```python
from build123d import *

# Parameters (mm, degrees)
SKETCH_1_W          = 82
SKETCH_1_H          = 40
EXTRUDE_1_DEPTH     = 8
SKETCH_3_W          = 10
SKETCH_3_H          = 5
EXTRUDE_3_DEPTH     = 20
SKETCH_4_R          = 1.5
CUT_EXTRUDE_1_DEPTH = 47


with BuildPart() as part:
    # 草图1 → 凸台-拉伸1 (new body)
    with BuildSketch(Plane.XY):
        with Locations((15.184210526, 10.907894737)):
            Rectangle(SKETCH_1_W, SKETCH_1_H)
        with BuildLine():
            Line((46.184210526, -1.592105263), (36.184210526, -1.592105263))
            ThreePointArc((36.184210526, -1.592105263), (33.684210526, 0.907894737), (36.184210526, 3.407894737))
            Line((36.184210526, 3.407894737), (46.184210526, 3.407894737))
            ThreePointArc((46.184210526, 3.407894737), (48.684210526, 0.907894737), (46.184210526, -1.592105263))
        make_face(mode=Mode.SUBTRACT)
        with BuildLine():
            Line((46.184210526, 18.407894737), (36.184210526, 18.407894737))
            ThreePointArc((36.184210526, 18.407894737), (33.684210526, 20.907894737), (36.184210526, 23.407894737))
            Line((36.184210526, 23.407894737), (46.184210526, 23.407894737))
            ThreePointArc((46.184210526, 23.407894737), (48.684210526, 20.907894737), (46.184210526, 18.407894737))
        make_face(mode=Mode.SUBTRACT)
    extrude(amount=EXTRUDE_1_DEPTH)

    # 草图3 → 凸台-拉伸3 (add)
    with BuildSketch(Plane.XY.offset(8)):
        with Locations((-20.815789474, 28.407894737)):
            Rectangle(SKETCH_3_W, SKETCH_3_H)
        with Locations((-20.815789474, -6.592105263)):
            Rectangle(SKETCH_3_W, SKETCH_3_H)
        with Locations((-20.815789474, 10.907894737)):
            Rectangle(SKETCH_3_W, SKETCH_3_H)
    extrude(amount=EXTRUDE_3_DEPTH)

    # 草图4 → 切除-拉伸1 (cut)
    with BuildSketch(Plane(origin=(0, 30.907894737, 0), x_dir=(1, 0, 0), z_dir=(0, 1, 0))):
        with Locations(Location((-20.815789474, -18, 0), (0, 0, 270))):
            Circle(SKETCH_4_R)
    extrude(amount=-CUT_EXTRUDE_1_DEPTH, mode=Mode.SUBTRACT)


solid = part.part
```
Geometry check sheet. Reference: the model listing, model coordinates, mm. A direction names the side the tool comes from. Give positions to 0.01 mm unless a question says otherwise; leave off trailing zeros. Write each loop counter-clockwise with the first axis right and the second up, starting at its lowest first coordinate (ties: lowest second). Pieces come first, ordered by that corner, then holes.
1) Section check C-C, the plane z = 18. Record the boundary of the cut face in (x, y), and give its area (3 significant figures).
2) Section check A-A, the plane z = 24.25. Record the boundary of the cut face in (x, y), and give its area (3 significant figures).
3) Gauge pin test, flat ends, axial feed: pin 1 (3 mm diameter, centred on x = 25, y = 10, fed in from -Z); pin 2 (4 mm diameter, centred on y = -6, z = 17, fed in from +X); pin 3 (5 mm diameter, centred on x = 41, y = 5.5, fed in from +Z). Record the tip position at first contact, or that the pin passes through.
4) Section check D-D, the plane y = 21.5. Record the boundary of the cut face in (x, z).
5) Material ranges on L1, parallel to Y at x = 46, z = 1.75; L2, parallel to X at y = 11.15, z = 18; L3, parallel to Z at x = -17, y = 6, recorded low to high.
6) Section check B-B, the plane x = 41. Record the boundary of the cut face in (y, z), and give its area (3 significant figures).
7) Access from +Z, -Z, +X, -X, +Y, -Y to the whole of each face (thin tool, end or side, straight path). Record for faces 1 (the flat face through (-19, 8.408, 18)), 2 (the cylindrical face through (33.685, 0.853, 3.944)), 3 (the flat face through (-15.816, 28, 18)).
8) Release check for a two-part mould opening along Y. For faces 4 (the flat face through (41, 18.408, 4)), 5 (the cylindrical face through (-20.75, 28.44, 16.5)), 6 (the flat face through (5.5, -9.092, 7.6)) record: pulls with the +Y half, pulls with the -Y half, needs draft (parallel to the pull), parting line crosses it, or undercut.
Computed:
1. outline: (-25.82, -9.09) - (-22.32, -9.09) - (-22.32, -4.09) - (-25.82, -4.09) - close; (-25.82, 8.41) - (-22.32, 8.41) - (-22.32, 13.41) - (-25.82, 13.41) - close; (-25.82, 25.91) - (-22.32, 25.91) - (-22.32, 30.91) - (-25.82, 30.91) - close; (-19.32, -9.09) - (-15.82, -9.09) - (-15.82, -4.09) - (-19.32, -4.09) - close; (-19.32, 8.41) - (-15.82, 8.41) - (-15.82, 13.41) - (-19.32, 13.41) - close; (-19.32, 25.91) - (-15.82, 25.91) - (-15.82, 30.91) - (-19.32, 30.91) - close
1. area: 105 mm2
2. outline: (-25.82, -9.09) - (-15.82, -9.09) - (-15.82, -4.09) - (-25.82, -4.09) - close; (-25.82, 8.41) - (-15.82, 8.41) - (-15.82, 13.41) - (-25.82, 13.41) - close; (-25.82, 25.91) - (-15.82, 25.91) - (-15.82, 30.91) - (-25.82, 30.91) - close
2. area: 150 mm2
3. pin 1: stops at z = 0
3. pin 2: stops at x = -15.82
3. pin 3: stops at z = 8
4. outline: (-25.82, 0) - (33.76, 0) - (33.76, 8) - (-25.82, 8) - close; (48.61, 0) - (56.18, 0) - (56.18, 8) - (48.61, 8) - close
5. L1: y = -9.09 to -1.59, 3.41 to 18.41, 23.41 to 30.91
5. L2: x = -25.82 to -22.32, -19.32 to -15.82
5. L3: z = 0 to 8
6. outline: (-9.09, 0) - (-1.59, 0) - (-1.59, 8) - (-9.09, 8) - close; (3.41, 0) - (18.41, 0) - (18.41, 8) - (3.41, 8) - close; (23.41, 0) - (30.91, 0) - (30.91, 8) - (23.41, 8) - close
6. area: 240 mm2
7. face 1: +Z, +X, -X
7. face 2: +Z, -Z
7. face 3: +Z, +X, +Y, -Y
8. face 4: undercut
8. face 5: needs draft
8. face 6: pulls with the -Y half
